Autodesk Inventor part; units mm, degrees
ref_plane "YZ Plane" through (0, 0, 0) normal (1, 0, 0) x (0, 1, 0)
ref_plane "XZ Plane" through (0, 0, 0) normal (0, 1, 0) x (-1, 0, 0)
ref_plane "XY Plane" through (0, 0, 0) normal (0, 0, 1) x (1, 0, 0)
sketch "Sketch1" plane through (0, 0, 0) normal (0, 0, 1) x (1, 0, 0)
  line L0 (0, 0) -> (0, 8.5)
  line L1 (0, 8.5) -> (8.5, 8.5)
  line L2 (8.5, 8.5) -> (8.5, -8.5)
  line L3 (8.5, -8.5) -> (-8.5, -8.5)
  line L4 (-8.5, -8.5) -> (-8.5, 8.5)
  line L5 (-8.5, 8.5) -> (0, 8.5)
  line L6 (0, 8.5) -> (0, 10.25)
  line L7 (0, 10.25) -> (-23.8, 10.25)
  line L8 (-23.8, 10.25) -> (-23.8, 6.92)
  circle A0 centre (-23.8, 6.92) radius 1.5
  line L9 (0, 10.25) -> (23.8, 10.25)
  line L10 (23.8, 10.25) -> (23.8, 6.92)
  circle A1 centre (23.8, 6.92) radius 1.5
  line L11 (-23.8, 6.92) -> (-23.8, -26.28)
  circle A2 centre (-23.8, -26.28) radius 1.5
  line L12 (0, 0) -> (0, 6.92)
  line L13 (-25.3, 6.92) -> (-26.55, 6.92)
  line L14 (-26.55, 6.92) -> (-26.55, -28.83)
  line L15 (-26.55, 6.92) -> (-26.55, 11.5)
  line L16 (-26.55, 11.5) -> (27.45, 11.5)
  line L17 (27.45, 11.5) -> (27.45, 11.5)
  line L18 (27.45, 11.5) -> (27.45, -28.83)
  line L19 (27.45, -28.83) -> (-26.55, -28.83)
  dimension "d8" = 3
  dimension "d0" = 8.5
  dimension "d1" = 8.5
  dimension "d2" = 17
  dimension "d3" = 17
  dimension "d4" = 17
  dimension "d5" = 1.75
  dimension "d6" = 23.8
  dimension "d7" = 3.33
  dimension "d9" = 23.8
  dimension "d10" = 3.33
  dimension "d11" = 3
  dimension "d12" = 33.2
  dimension "d13" = 3
  dimension "d14" = 1.25
  dimension "d15" = 35.75
  dimension "d16" = 4.58
  dimension "d17" = 0
  dimension "d33" = 54
extrude "Extrusion1" add sketch "Sketch1" along normal blind 1.65
sketch "Sketch2" plane through (0, 0, 1.65) normal (0, 0, 1) x (1, 0, 0)
  line L0 (-8.5, 8.5) -> (-8.5, -8.5)
  line L1 (8.5, 8.5) -> (8.5, -8.5)
  line L2 (-8.5, 8.5) -> (8.5, 8.5)
  line L3 (8.5, 8.5) -> (8.5, -8.5)
  line L4 (8.5, -8.5) -> (-8.5, -8.5)
  line L5 (-8.5, -8.5) -> (-8.5, 8.5)
  point P0 (0, 0)
extrude "Extrusion2" add sketch "Sketch2" along normal blind 8 and the other way blind 1.65
sketch "Sketch3" plane through (0, 0, 9.65) normal (0, 0, 1) x (1, 0, 0)
  circle A0 centre (0, 0) radius 7.5
  dimension "d24" = 15
extrude "Extrusion3" add sketch "Sketch3" along normal blind 16
sketch "Sketch4" plane through (0, 0, 1.65) normal (0, 0, 1) x (1, 0, 0)
  line L0 (-26.55, -28.83) -> (27.45, -28.83)
  line L1 (-26.55, -28.83) -> (27.45, -28.83)
  line L2 (27.45, -28.83) -> (27.45, -34.38)
  line L3 (27.45, -34.38) -> (-26.55, -34.38)
  line L4 (-26.55, -34.38) -> (-26.55, -28.83)
  point P0 (0, 0)
  dimension "d27" = 5.55
  dimension "d34" = 54
extrude "Extrusion4" add sketch "Sketch4" against normal blind 1.65
sketch "Sketch5" plane through (0, 0, 1.65) normal (0, 0, 1) x (1, 0, 0)
  line L0 (27.45, -34.38) -> (-26.55, -34.38)
  line L1 (-26.55, -34.38) -> (-13.95, -34.38)
  line L2 (-13.95, -34.38) -> (-13.95, -40.78)
  line L3 (-13.95, -40.78) -> (14.65, -40.78)
  line L4 (14.65, -40.78) -> (14.65, -34.38)
  line L5 (14.65, -34.38) -> (-13.95, -34.38)
  point P0 (0, 0)
  dimension "d30" = 12.6
  dimension "d31" = 6.4
  dimension "d32" = 28.6
extrude "Extrusion5" add sketch "Sketch5" against normal blind 1.65
equation "\"d9\" = d6"
properties part number "Pixy Sketch"
Here's how the part is built. I have some questions about the finished solid (model axes, mm). A direction names the side the tool comes from. Give positions to 0.01 mm unless a question says otherwise; leave off trailing zeros. Write each loop counter-clockwise with the first axis right and the second up, starting at its lowest first coordinate (ties: lowest second). Pieces come first, ordered by that corner, then holes. Notation, with made-up numbers: (30, -24) -> (57, -24) arc R12 cw to (57, -11) -> close; hole circle Ø2 at (-4, 59). An arc over 180 degrees is marked (long way). Use one line per item in the form item = value.
1) Suppose I cut it at D-D (z = 22). Please give me the cut outline in (x, y).
Verdict:
outline = circle Ø15 at (0, 0)
2) Suppose I cut it at C-C (y = 0). Please give me the cut outline in (x, z), and give its area (3 significant figures).
Verdict:
outline = (-26.55, 0) -> (27.45, 0) -> (27.45, 1.65) -> (8.5, 1.65) -> (8.5, 9.65) -> (7.5, 9.65) -> (7.5, 25.65) -> (-7.5, 25.65) -> (-7.5, 9.65) -> (-8.5, 9.65) -> (-8.5, 1.65) -> (-26.55, 1.65) -> close
area = 465 mm2
3) If I drill on L1, parallel to Y at x = -23.8, z = 1.2; L2, parallel to Y at x = 23.8, z = 0.9; L3, parallel to Z at x = 1, y = -19, over which ranges is the centre line in solid material (lowest first)? Write a range as [from, to].
Verdict:
L1 = [-34.38, -27.78], [-24.78, 5.42], [8.42, 11.5]
L2 = [-34.38, 5.42], [8.42, 11.5]
L3 = [0, 1.65]
4) On a 3-axis mill with a long thin cutter (end or side, diameter ignored), from which of +Z, -Z, +X, -X, +Y, -Y can I reach the whole of each face in a straight line? I mean faces 5 (the face through (-7.493, -0.33, 17.538)), 6 (the face through (-8.5, 0, 6)), 7 (the face through (0, -8.5, 6)), 8 (the face through (-20, -34.38, 1)). Say none if no direction works.
Verdict:
face_5 = +Z
face_6 = +Z, -X, +Y, -Y
face_7 = +Z, +X, -X, -Y
face_8 = +Z, -Z, -X, -Y
5) We'd pull the mould along X, two halves only. Please class faces 1 (the face through (21, -34.38, 1)), 2 (the face through (-24.99, 7.83, 0.81)), 3 (the face through (-26.55, -12, 1)), 4 (the face through (14.65, -38, 1)): +X half, -X half, draft (parallel to the pull), parting line (faces both ways), or undercut.
Verdict:
face_1 = draft
face_2 = undercut
face_3 = -X half
face_4 = +X half
6) Suppose I cut it at A-A (x = 23.8). Please give me the cut outline in (y, z).
Verdict:
outline = (-34.38, 0) -> (5.42, 0) -> (5.42, 1.65) -> (-34.38, 1.65) -> close; (8.42, 0) -> (11.5, 0) -> (11.5, 1.65) -> (8.42, 1.65) -> close
7) I'm going to push flat-ended pins straight in: pin 1 (5 mm diameter, centred on x = 3, y = -18, fed in from +Z); pin 2 (0.8 mm diameter, centred on y = -38.5, z = 1, fed in from -X); pin 3 (1 mm diameter, centred on y = 1, z = 21.5, fed in from +X). Where does each tip first touch, or does it pass through?
Verdict:
pin_1 = 1.65
pin_2 = -13.95
pin_3 = 7.48
8) Suppose I cut it at B-B (y = -26.28). Please give me the cut outline in (x, z), and give its area (4 significant figures).
Verdict:
outline = (-26.55, 0) -> (-25.3, 0) -> (-25.3, 1.65) -> (-26.55, 1.65) -> close; (-22.3, 0) -> (27.45, 0) -> (27.45, 1.65) -> (-22.3, 1.65) -> close
area = 84.15 mm2
